from build123d import *

# Parameters (mm, degrees)
SKETCH1_R                                    = 1.5
SKETCH1_R_2                                  = 3
BOSS_EXTRUDE1_DEPTH                          = 1.5
CSK_FOR_M1_6_COUNTERSUNK_FLAT_HEAD_S_2_COUNT = 2
CSK_FOR_M1_6_COUNTERSUNK_FLAT_HEAD_S_2_PITCH = 15.5
CSK_FOR_M1_6_COUNTERSUNK_FLAT_HEAD_S_3_COUNT = 2
CSK_FOR_M1_6_COUNTERSUNK_FLAT_HEAD_S_3_PITCH = 65.25
CSK_FOR_M1_6_COUNTERSUNK_FLAT_HEAD_S_4_COUNT = 2
CSK_FOR_M1_6_COUNTERSUNK_FLAT_HEAD_S_4_PITCH = 57.75


with BuildPart() as part:
    # Sketch1 → Boss-Extrude1 (new body)
    with BuildSketch(Plane.XY):
        with BuildLine():
            Line((15.5, 5.5), (-62, 5.5))
            ThreePointArc((-62, 5.5), (-67.5, 0), (-62, -5.5))
            Line((-62, -5.5), (15.5, -5.5))
            ThreePointArc((15.5, -5.5), (21, 0), (15.5, 5.5))
        make_face()
        with Locations((-62, 0)):
            Circle(SKETCH1_R, mode=Mode.SUBTRACT)
        Circle(SKETCH1_R_2, mode=Mode.SUBTRACT)
        with Locations((15.5, 0)):
            Circle(SKETCH1_R_2, mode=Mode.SUBTRACT)
    extrude(amount=BOSS_EXTRUDE1_DEPTH)

    # Sketch2 → CSK for M1.6 Countersunk Flat Head Screw1 (revolve, cut)
    with BuildSketch(Plane(origin=(7.75, 2.5, 1.5), x_dir=(0, -1, 0), z_dir=(1, 0, 0))):
        Polygon((0, 0), (0, 1.5), (0.9, 1.5), (0.9, 0.9), (1.8, 0), align=None)
    csk_for_m1_6_countersunk_flat_head_screw = revolve(axis=Axis((7.75, 2.5, 7.85), (0, 0, -1)), mode=Mode.SUBTRACT)

    # CSK for M1.6 Countersunk Flat Head S 2: CSK for M1.6 Countersunk Flat Head Screw1 ×2
    with Locations(*[(-i * CSK_FOR_M1_6_COUNTERSUNK_FLAT_HEAD_S_2_PITCH, 0, 0) for i in range(1, CSK_FOR_M1_6_COUNTERSUNK_FLAT_HEAD_S_2_COUNT)]):
        add(csk_for_m1_6_countersunk_flat_head_screw, mode=Mode.SUBTRACT)

    # CSK for M1.6 Countersunk Flat Head S 3: CSK for M1.6 Countersunk Flat Head Screw1 ×2
    with Locations(*[(-i * CSK_FOR_M1_6_COUNTERSUNK_FLAT_HEAD_S_3_PITCH, 0, 0) for i in range(1, CSK_FOR_M1_6_COUNTERSUNK_FLAT_HEAD_S_3_COUNT)]):
        add(csk_for_m1_6_countersunk_flat_head_screw, mode=Mode.SUBTRACT)

    # CSK for M1.6 Countersunk Flat Head S 4: CSK for M1.6 Countersunk Flat Head Screw1 ×2
    with Locations(*[(-i * CSK_FOR_M1_6_COUNTERSUNK_FLAT_HEAD_S_4_PITCH, 0, 0) for i in range(1, CSK_FOR_M1_6_COUNTERSUNK_FLAT_HEAD_S_4_COUNT)]):
        add(csk_for_m1_6_countersunk_flat_head_screw, mode=Mode.SUBTRACT)

    # Mirror1: CSK for M1.6 Countersunk Flat Head Screw1 across plane
    add(csk_for_m1_6_countersunk_flat_head_screw.mirror(Plane.ZX), mode=Mode.SUBTRACT)

    # Mirror1 copy 1 sketch → Mirror1 copy 1 (revolve, cut)
    with BuildSketch(Plane(origin=(-7.75, -2.5, 1.5), x_dir=(0, 1, 0), z_dir=(1, 0, 0))):
        Polygon((0, 0), (0, -1.5), (0.9, -1.5), (0.9, -0.9), (1.8, 0), align=None)
    revolve(axis=Axis((-7.75, -2.5, 7.85), (0, 0, 1)), mode=Mode.SUBTRACT)

    # Mirror1 copy 2 sketch → Mirror1 copy 2 (revolve, cut)
    with BuildSketch(Plane(origin=(-57.5, -2.5, 1.5), x_dir=(0, 1, 0), z_dir=(1, 0, 0))):
        Polygon((0, 0), (0, -1.5), (0.9, -1.5), (0.9, -0.9), (1.8, 0), align=None)
    revolve(axis=Axis((-57.5, -2.5, 7.85), (0, 0, 1)), mode=Mode.SUBTRACT)

    # Mirror1 copy 3 sketch → Mirror1 copy 3 (revolve, cut)
    with BuildSketch(Plane(origin=(-50, -2.5, 1.5), x_dir=(0, 1, 0), z_dir=(1, 0, 0))):
        Polygon((0, 0), (0, -1.5), (0.9, -1.5), (0.9, -0.9), (1.8, 0), align=None)
    revolve(axis=Axis((-50, -2.5, 7.85), (0, 0, 1)), mode=Mode.SUBTRACT)


solid = part.part
Geometry check sheet. Reference: the model listing, model coordinates, mm. Round coordinates to 2 decimals unless told otherwise and drop trailing zeros. Write each loop counter-clockwise with the first axis right and the second up, starting at its lowest first coordinate (ties: lowest second). Pieces come first, ordered by that corner, then holes. Notation, with made-up numbers: (42, 89) -> (85, 89) arc R20 ccw to (85, 105) -> close; hole circle Ø10 at (-29, 16). An arc over 180 degrees is marked (long way). One line per item, written item: value. Start each with the question number.
(1) Draft check along X on faces 1 (the cylindrical face through (21, 0, 1)), 2 (the cylindrical face through (-49.121, 2.695, 0.304)), 3 (the flat face through (-24, -5.5, 1)). Enter one of: +X half, -X half, draft (parallel to the pull), parting line (faces both ways), or undercut.
(2) Go/stop test with flat-tipped pins: pin 1 Ø2 at (x, y) = (-7.75, 2.5) entering from +Z; pin 2 Ø1.6 at (x, y) = (7.75, -2.5) entering from +Z; pin 3 Ø2.5 at (x, y) = (-7.75, -2.5) entering from +Z. Record where each tip stops, or that it passes through.
(3) Cross-section at A-A, the plane x = -7.75. Record the cut outline in (y, z), and give its area (3 significant figures).
(4) Scan lines: line 1 (Y direction, x = -50, z = 0.55); line 2 (Y direction, x = 15.5, z = 1.1); line 3 (Y direction, x = 7, z = 0.2). Record each from-to range of solid material in increasing order. Write a range as [from, to].
(5) Cross-section at B-B, the plane z = 0.25. Give the number of separate pieces and of enclosed holes in the cut face, and give its area (3 significant figures).
Answer:
1. face 1: +X half
1. face 2: undercut
1. face 3: draft
2. pin 1: z = 0.7
2. pin 2: through
2. pin 3: z = 0.95
3. outline: (-5.5, 0) -> (-3.4, 0) -> (-3.4, 0.6) -> (-4.3, 1.5) -> (-5.5, 1.5) -> close; (-1.6, 0) -> (1.6, 0) -> (1.6, 0.6) -> (0.7, 1.5) -> (-0.7, 1.5) -> (-1.6, 0.6) -> close; (3.4, 0) -> (5.5, 0) -> (5.5, 1.5) -> (4.3, 1.5) -> (3.4, 0.6) -> close
3. area: 9.48 mm²
4. line 1: [-5.5, -3.4], [-1.6, 1.6], [3.4, 5.5]
4. line 2: [-5.5, -3], [3, 5.5]
4. line 3: [-5.5, -3], [-2, 2], [3, 5.5]
5. separate pieces: 1
5. enclosed holes: 11
5. area: 864 mm²
